Here's the drawing with two shaded views (mm, measured from the low corner). I have some questions. A direction names the side the tool comes from. Coordinates: 2 decimals unless noted, no trailing zeros. Write each loop counter-clockwise with the first axis right and the second up, starting at its lowest first coordinate (ties: lowest second). Pieces come first, ordered by that corner, then holes.
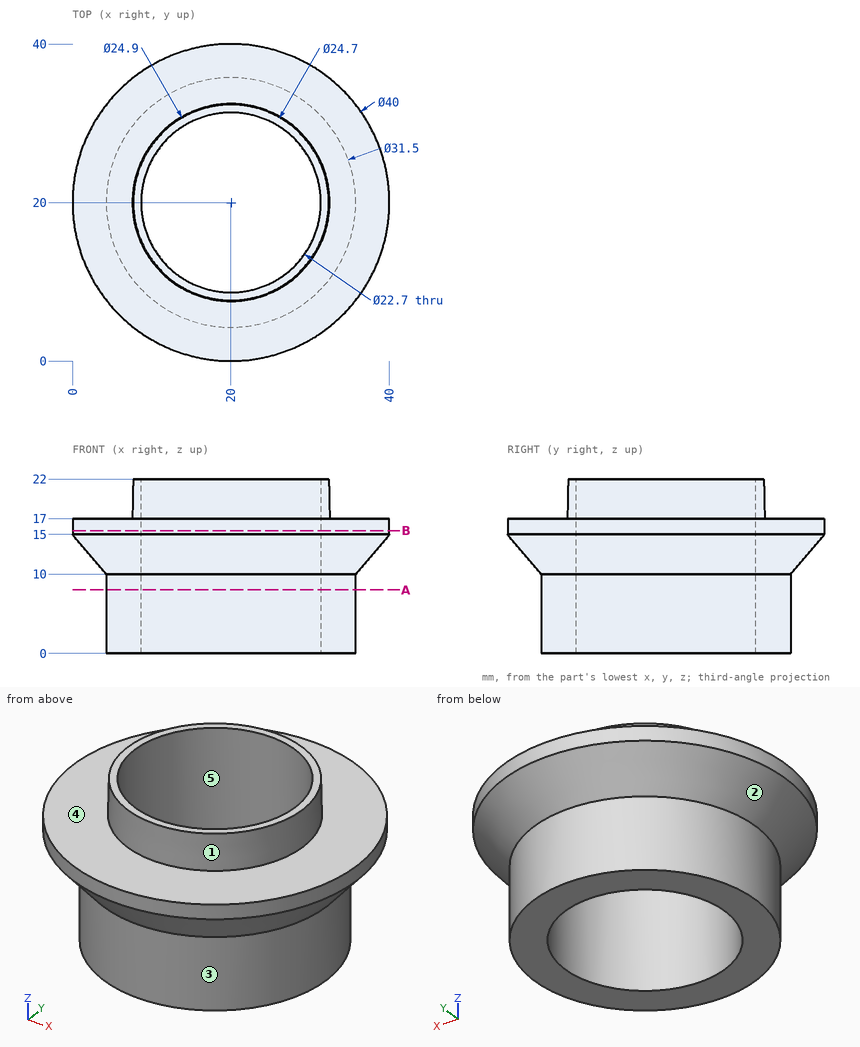
1. On a 3-axis mill with a long thin cutter (end or side, diameter ignored), from which of +Z, -Z, +X, -X, +Y, -Y can I reach the whole of each face in a straight line? I mean the marked faces 1 and 2. Say none if no direction works.
Verdict:
face 1: +Z
face 2: -Z
2. If we mould it in two halves opening along X, with no side actions, what happens to the marked faces 3, 4 and 5? For each: pulls with the +X half, pulls with the -X half, needs draft (parallel to the pull), parting line crosses it, or undercut.
Verdict:
face 3: parting line crosses it
face 4: needs draft
face 5: undercut
3. I want a section at A-A on z = 8. Please give me the cut outline in (x, y).
Verdict:
outline: circle Ø31.5 at (20, 20); hole circle Ø22.7 at (20, 20)
4. Please list where these lines run through material, in increasing order: line 1 along Y through (x, z) = (20, 6.25); line 2 along Y through (x, z) = (20, 15); line 3 along Z through (x, y) = (31, 30).
Verdict:
line 1: y = 4.25 to 8.65, 31.35 to 35.75
line 2: y = 0 to 8.65, 31.35 to 40
line 3: z = 0 to 17
5. For pin 1 (12 mm diameter, centred on x = 12.5, z = 6.5, fed in from +Y); pin 2 (6 mm diameter, centred on x = 30, y = 35.5, fed in from +Z); pin 3 (4 mm diameter, centred on x = 12.5, z = 13, fed in from -Y), each with a flat end and sliding along its axis, tell me the tip position at first contact or that it passes through.
Verdict:
pin 1: stops at y = 36.7
pin 2: stops at z = 17
pin 3: stops at y = 1.31
6. I want a section at B-B on z = 15.5. Please give me the cut outline in (x, y).
Verdict:
outline: circle Ø40 at (20, 20); hole circle Ø22.7 at (20, 20)
